```python
from build123d import *

# Parameters (mm, degrees)
SKETCH1_R           = 1.5
BOSS_EXTRUDE1_DEPTH = 5
BOSS_EXTRUDE2_DEPTH = 10
SKETCH3_R           = 4
CUT_EXTRUDE1_DEPTH  = 4
SKETCH3_3_R         = 3
CUT_EXTRUDE2_DEPTH  = 45.102862719
FILLET6_R           = 3.5
FILLET7_R           = 3.5
FILLET8_R           = 3.5
FILLET9_R           = 3.5
FILLET10_R          = 3.5
FILLET11_R          = 3.5
FILLET12_R          = 1
FILLET13_R          = 1
FILLET14_R          = 1
FILLET15_R          = 1
FILLET16_R          = 1
FILLET17_R          = 1
FILLET18_R          = 1
FILLET19_R          = 1
SKETCH4_W           = 15
SKETCH4_H           = 5.75
CUT_EXTRUDE3_DEPTH  = 32.305949934
SKETCH5_W           = 24
SKETCH5_H           = 12.5
SKETCH5_W_2         = 15
SKETCH5_H_2         = 5.75
CUT_EXTRUDE4_DEPTH  = 2


with BuildPart() as part:
    # Sketch1 → Boss-Extrude1 (new body)
    with BuildSketch(Plane(origin=(0, 0, 0), x_dir=(1, 0, 0), z_dir=(0, 1, 0))):
        with BuildLine():
            Line((-25, -4), (-25, -6.25))
            Line((-25, -6.25), (25, -6.25))
            Line((25, -6.25), (25, -4))
            ThreePointArc((25, -4), (29, 0), (25, 4))
            Line((25, 4), (25, 6.25))
            Line((25, 6.25), (-25, 6.25))
            Line((-25, 6.25), (-25, 4))
            ThreePointArc((-25, 4), (-29, 0), (-25, -4))
        make_face()
        with Locations(Location((25, 0, 0), (0, 0, 270))):
            Circle(SKETCH1_R, mode=Mode.SUBTRACT)
        with Locations(Location((-25, 0, 0), (0, 0, 270))):
            Circle(SKETCH1_R, mode=Mode.SUBTRACT)
    extrude(amount=BOSS_EXTRUDE1_DEPTH)

    # Sketch2 → Boss-Extrude2 (add)
    with BuildSketch(Plane(origin=(0, 5, 0), x_dir=(1, 0, 0), z_dir=(0, 1, 0))):
        Polygon((-18, 0), (-18, -6.25), (-12, -6.25), (-12, 6.25), (-18, 6.25), align=None)
    boss_extrude2 = extrude(amount=BOSS_EXTRUDE2_DEPTH)

    # Sketch3 → Cut-Extrude1 (cut)
    with BuildSketch(Plane(origin=(-12, 0, 0), x_dir=(0, 0, -1), z_dir=(1, 0, 0))):
        with Locations((0, 10)):
            Circle(SKETCH3_R)
    cut_extrude1 = extrude(amount=-CUT_EXTRUDE1_DEPTH, mode=Mode.SUBTRACT)

    # Sketch3<3> → Cut-Extrude2 (cut, through all)
    with BuildSketch(Plane(origin=(-12, 0, 0), x_dir=(0, 0, -1), z_dir=(1, 0, 0))):
        with Locations((0, 10)):
            Circle(SKETCH3_3_R)
    cut_extrude2 = extrude(amount=-CUT_EXTRUDE2_DEPTH, mode=Mode.SUBTRACT)

    # Fillet6
    # the kernel refuses this fillet: 3.5 mm, written as the material it adds along each edge
    with BuildSketch(Plane(origin=(-18, 5, -6.25), x_dir=(0, 1, 0), z_dir=(0, 0, 1))) as fillet6_piece_1_section:
        with BuildLine():
            CenterArc((FILLET6_R, FILLET6_R), FILLET6_R, 180, 90)
            Line((0, FILLET6_R), (0, 0))
            Line((0, 0), (FILLET6_R, 0))
        make_face()
    fillet6_piece_1 = extrude(amount=12.5, mode=Mode.PRIVATE)
    fillet6_piece_1 = fillet6_piece_1 - Plane(origin=(-18.808785758, 10, 0), x_dir=(0, 0, -1), z_dir=(1, 0, 0)) * Cylinder(3, 39, mode=Mode.PRIVATE)
    add(fillet6_piece_1)

    # Fillet7
    fillet7_edges = [part.edges().sort_by_distance(p)[0] for p in [
        (-15, 15, -6.25),
    ]]
    fillet(fillet7_edges, radius=FILLET7_R)

    # Fillet8
    fillet8_edges = [part.edges().sort_by_distance(p)[0] for p in [
        (-15, 15, 6.25),
    ]]
    fillet(fillet8_edges, radius=FILLET8_R)

    # Mirror4: Boss-Extrude2, Cut-Extrude1, Cut-Extrude2 across plane
    add(boss_extrude2.mirror(Plane(origin=(0, 0, 0), x_dir=(0, 0, 1), z_dir=(1, 0, 0))))
    add(cut_extrude1.mirror(Plane(origin=(0, 0, 0), x_dir=(0, 0, 1), z_dir=(1, 0, 0))), mode=Mode.SUBTRACT)
    add(cut_extrude2.mirror(Plane(origin=(0, 0, 0), x_dir=(0, 0, 1), z_dir=(1, 0, 0))), mode=Mode.SUBTRACT)

    # Fillet9
    fillet9_edges = [part.edges().sort_by_distance(p)[0] for p in [
        (15, 15, -6.25),
    ]]
    fillet(fillet9_edges, radius=FILLET9_R)

    # Fillet10
    fillet10_edges = [part.edges().sort_by_distance(p)[0] for p in [
        (15, 15, 6.25),
    ]]
    fillet(fillet10_edges, radius=FILLET10_R)

    # Fillet11
    # the kernel refuses this fillet: 3.5 mm, written as the material it adds along each edge
    with BuildSketch(Plane(origin=(18, 5, -6.25), x_dir=(0, 1, 0), z_dir=(0, 0, 1))) as fillet11_piece_1_section:
        with BuildLine():
            CenterArc((FILLET11_R, -FILLET11_R), FILLET11_R, 90, 90)
            Line((0, -FILLET11_R), (0, 0))
            Line((0, 0), (FILLET11_R, 0))
        make_face()
    fillet11_piece_1 = extrude(amount=12.5, mode=Mode.PRIVATE)
    fillet11_piece_1 = fillet11_piece_1 - Plane(origin=(18.808785758, 10, 0), x_dir=(0, 0, -1), z_dir=(-1, 0, 0)) * Cylinder(3, 39, mode=Mode.PRIVATE)
    add(fillet11_piece_1)

    # Fillet12
    fillet12_edges = [part.edges().sort_by_distance(p)[0] for p in [
        (25, 2.5, -6.25),
    ]]
    fillet(fillet12_edges, radius=FILLET12_R)

    # Fillet13
    fillet13_edges = [part.edges().sort_by_distance(p)[0] for p in [
        (25, 2.5, 6.25),
    ]]
    fillet(fillet13_edges, radius=FILLET13_R)

    # Fillet14
    fillet14_edges = [part.edges().sort_by_distance(p)[0] for p in [
        (-25, 2.5, 6.25),
    ]]
    fillet(fillet14_edges, radius=FILLET14_R)

    # Fillet15
    fillet15_edges = [part.edges().sort_by_distance(p)[0] for p in [
        (-25, 2.5, -6.25),
    ]]
    fillet(fillet15_edges, radius=FILLET15_R)

    # Fillet16
    fillet16_edges = [part.edges().sort_by_distance(p)[0] for p in [
        (-25, 2.5, -4),
    ]]
    fillet(fillet16_edges, radius=FILLET16_R)

    # Fillet17
    fillet17_edges = [part.edges().sort_by_distance(p)[0] for p in [
        (-25, 2.5, 4),
    ]]
    fillet(fillet17_edges, radius=FILLET17_R)

    # Fillet18
    fillet18_edges = [part.edges().sort_by_distance(p)[0] for p in [
        (25, 2.5, 4),
    ]]
    fillet(fillet18_edges, radius=FILLET18_R)

    # Fillet19
    fillet19_edges = [part.edges().sort_by_distance(p)[0] for p in [
        (25, 2.5, -4),
    ]]
    fillet(fillet19_edges, radius=FILLET19_R)

    # Sketch4 → Cut-Extrude3 (cut, through all)
    with BuildSketch(Plane(origin=(0, 5, 0), x_dir=(1, 0, 0), z_dir=(0, 1, 0))):
        Rectangle(SKETCH4_W, SKETCH4_H)
    extrude(amount=-CUT_EXTRUDE3_DEPTH, mode=Mode.SUBTRACT)

    # Sketch5 → Cut-Extrude4 (cut)
    with BuildSketch(Plane(origin=(0, 5, 0), x_dir=(1, 0, 0), z_dir=(0, 1, 0))):
        Rectangle(SKETCH5_W, SKETCH5_H)
        Rectangle(SKETCH5_W_2, SKETCH5_H_2, mode=Mode.SUBTRACT)
    extrude(amount=-CUT_EXTRUDE4_DEPTH, mode=Mode.SUBTRACT)


solid = part.part
```
Geometry check sheet. Reference: the model listing, model coordinates, mm. A direction names the side the tool comes from. Round coordinates to 2 decimals unless told otherwise and drop trailing zeros. Order: outer loops, then holes, each group sorted by start corner. A loop starts at its lowest first (then second) coordinate and runs counter-clockwise, first axis right, second up. Notation, with made-up numbers: (71.5, -15.75) - (108.5, -15.75) arc R10 ccw to (108.5, -10.75) - close; hole circle Ø2 at (-19.5, 53.5). An arc over 180 degrees is marked (long way). Use a Markdown table: item, result. Add a question column.
(1) Depth check by flat-ended pin: pin 1 (1 mm diameter, centred on x = -19.5, z = 0.5, fed in from +Y); pin 2 (4 mm diameter, centred on y = 12.5, z = -3.5, fed in from -X); pin 3 (2 mm diameter, centred on y = 13, z = -3, fed in from +X); pin 4 (2.5 mm diameter, centred on x = 25, z = 0, fed in from +Y). Enter the tip coordinate at first touch or a pass-through.
(2) Release check for a two-part mould opening along X. For faces 1 (the cylindrical face through (-15, 14, 5.2)), 2 (the cylindrical face through (-19.05, 6, -0.09)), 3 (the flat face through (-7.5, 2, 0)), 4 (the cylindrical face through (-13.972, 13.966, 0.521)) record: pulls with the +X half, pulls with the -X half, needs draft (parallel to the pull), parting line crosses it, or undercut.
(3) Sectioned sample at C-C, the plane z = 0. Count the separate pieces of the cut face and the enclosed holes in it, and give its area (3 significant figures).
(4) Sectioned sample at A-A, the plane y = 10. Enter the section's corners in (x, z), and give its area (3 significant figures).
(5) Material ranges on line 1 along X through (y, z) = (14, 3.5); line 2 along X through (y, z) = (11.5, -3); line 3 along Z through (x, y) = (-17.55, 10), recorded low to high. Write a range as [from, to].
(6) Tool access check on faces 5 (the flat face through (7.5, 2, 0)), 6 (the flat face through (-18, 13.15, -0.09)), 7 (the flat face through (-16, 13, -1)). Record the directions out of +Z, -Z, +X, -X, +Y, -Y that give a thin tool (end or side, any length) a straight path to the whole face; none if there is none.
(7) Sectioned sample at D-D, the plane x = -10. Enter the section's corners in (y, z).
(8) Sectioned sample at B-B, the plane x = 2. Enter the section's corners in (y, z) (3 decimals).
Answers below:
| question | item | result |
|---|---|---|
| 1 | pin 1 | y = 6.05 |
| 1 | pin 2 | x = -18 |
| 1 | pin 3 | x = 18 |
| 1 | pin 4 | through |
| 2 | face 1 | needs draft |
| 2 | face 2 | pulls with the -X half |
| 2 | face 3 | undercut |
| 2 | face 4 | undercut |
| 3 | separate pieces | 6 |
| 3 | enclosed holes | 0 |
| 3 | area | 204 mm² |
| 4 | outline | (-18, -6.25) - (-12, -6.25) - (-12, -4) - (-16, -4) - (-16, -3) - (-18, -3) - close; (-18, 3) - (-16, 3) - (-16, 4) - (-12, 4) - (-12, 6.25) - (-18, 6.25) - close; (12, -6.25) - (18, -6.25) - (18, -3) - (16, -3) - (16, -4) - (12, -4) - close; (12, 4) - (16, 4) - (16, 3) - (18, 3) - (18, 6.25) - (12, 6.25) - close |
| 4 | area | 62.0 mm² |
| 5 | line 1 | [-18, -12], [12, 18] |
| 5 | line 2 | [-18, -16], [16, 18] |
| 5 | line 3 | [-6.25, -3], [3, 6.25] |
| 6 | face 5 | +Y, -Y |
| 6 | face 6 | +Z, -Z, -X, +Y |
| 6 | face 7 | none |
| 7 | outline | (0, -6.25) - (3, -6.25) - (3, 6.25) - (0, 6.25) - close |
| 8 | outline | (0, -6.25) - (3, -6.25) - (3, -2.875) - (0, -2.875) - close; (0, 2.875) - (3, 2.875) - (3, 6.25) - (0, 6.25) - close |
